Autodesk Inventor part; units mm, degrees
ref_plane "YZ Plane" through (0, 0, 0) normal (1, 0, 0) x (0, 1, 0)
ref_plane "XZ Plane" through (0, 0, 0) normal (0, 1, 0) x (-1, 0, 0)
ref_plane "XY Plane" through (0, 0, 0) normal (0, 0, 1) x (1, 0, 0)
sketch "Sketch1" plane through (0, 0, 0) normal (0, 1, 0) x (-1, 0, 0)
  line L0 (10, -25) -> (10, 25)
  line L1 (-10, 25) -> (-10, -25)
  arc A0 (10, 25) -> (-10, 25) centre (0, 25) ccw
  arc A1 (-10, -25) -> (10, -25) centre (0, -25) ccw
  circle A2 centre (0, 25) radius 5
  circle A3 centre (0, -25) radius 5
  point P0 (0, 0)
extrude "Extrusion1" add sketch "Sketch1" along normal blind 50
sketch "Sketch2" plane through (-10, 0, -25) normal (-1, 0, 0) x (0, 0, 1)
  line L0 (-10, 0) -> (-10, 50)
  line L1 (10, 5) -> (-10, 5)
  line L2 (-10, 5) -> (-10, 45)
  line L3 (-10, 45) -> (10, 45)
  line L4 (10, 45) -> (10, 5)
  line L5 (0, 0) -> (0, 50)
  point P0 (25, 0)
  dimension "d6" = 40
extrude "Extrusion2" cut sketch "Sketch2" against normal up to surface (20 mm away)
mirror "Mirror1" about plane through (0, 0, 0) normal (0, 0, 1) of "Extrusion2"
fillet "Fillet1" radius 2 24 edges at (0, 50, -35) (-10, 50, 0) (0, 50, 35) (10, 50, 0) (0, 45, -35) (-10, 45, -20) (10, 45, -20) (10, 25, -15) (10, 25, 15) (10, 45, 20) (-10, 45, 20) (0, 45, 35) (-10, 25, 15) (-10, 5, 20) (10, 5, 20) (0, 5, 35) (10, 0, 0) (0, 0, -35) (-10, 0, 0) (0, 0, 35) (10, 5, -20) (-10, 5, -20) (0, 5, -35) (-10, 25, -15)
properties part number "Link2"
Check sheet for the modelled part. Datum: model origin and axes. Units: mm. A direction names the side the tool comes from. Coordinates: 2 decimals unless noted, no trailing zeros. Order: outer loops, then holes, each group sorted by start corner. A loop starts at its lowest first (then second) coordinate and runs counter-clockwise, first axis right, second up. Notation, with made-up numbers: M 13,0.5 L 19,0.5 A16 cw 19,25.5 Z; hole C 28,-15 d9. An arc over 180 degrees is marked long. Write each question's results on one line, items separated by ' | '. Start each with the question number.
1. Material ranges on probe 1 along Z at (x, y) = (0, 2.9); probe 2 along Y at (x, z) = (1.75, 17); probe 3 along Z at (x, y) = (3.75, 47.5), recorded low to high.
2. Access from +Z, -Z, +X, -X, +Y, -Y to the whole of each face (thin tool, end or side, straight path). Record for faces 5 (the face through (0, 25, 15)), 6 (the face through (9.4, 4.43, 18.92)), 7 (the face through (-9.4, 45.57, 18.92)), 8 (the face through (-2, 5, -20)), 9 (the face through (1.08, 47.46, -20.12)).
3. Cross-section at C-C on y = 9. Record the cut outline in (x, z).
4. Cross-section at A-A on z = 18.5. Record the cut outline in (x, y).
5. Go/stop test with flat-tipped pins: P1, Ø6, axis at x = -0.5, y = 45, coming from the -Z side; P2, Ø3, axis at x = -1, y = 13, coming from the -Z side; P3, Ø5, axis at x = -4, y = 17, coming from the +Z side. Record where each tip stops, or that it passes through.
6. Cross-section at B-B on x = 0. State how many separate pieces and enclosed holes the cut face has, and give its area (3 significant figures).
7. Mould release check, pull along Y, two halves, no side actions. Record for faces 1 (the face through (0, 50, 0)), 2 (the face through (1.08, 2.46, 29.88)), 3 (the face through (0, 25, -15)), 4 (the face through (9.43, 24.69, 14.4)): +Y half, -Y half, draft (parallel to the pull), parting line (faces both ways), or undercut.
Checks:
1) probe 1: z = -35 to -30, -20 to 20, 30 to 35 | probe 2: y = 0 to 5, 45 to 50 | probe 3: z = -34.27 to -28.31, -21.69 to 21.69, 28.31 to 34.27
2) face 5: +Z, +X, -X | face 6: +Z, +X | face 7: +Z, -X | face 8: -Z, +X, -X | face 9: +Y, -Y
3) outline: M -10,-13 A2 ccw -8,-15 L 8,-15 A2 ccw 10,-13 L 10,13 A2 ccw 8,15 L -8,15 A2 ccw -10,13 Z
4) outline: M -10,2 A2 ccw -8,0 L 8,0 A2 ccw 10,2 L 10,3 A2 ccw 8,5 L -8,5 A2 ccw -10,3 Z; M -10,47 A2 ccw -8,45 L 8,45 A2 ccw 10,47 L 10,48 A2 ccw 8,50 L -8,50 A2 ccw -10,48 Z
5) P1: stops at z = -35 | P2: stops at z = -15 | P3: stops at z = 15
6) separate pieces: 5 | enclosed holes: 0 | area: 1,690 mm²
7) face 1: +Y half | face 2: draft | face 3: undercut | face 4: undercut
